The listing builds one solid part. Answer for the finished solid, in the listing's coordinates (mm). Coordinates: 2 decimals unless noted, no trailing zeros. Order: outer loops, then holes, each group sorted by start corner. A loop starts at its lowest first (then second) coordinate and runs counter-clockwise, first axis right, second up.
from build123d import *

# Parameters (mm, degrees)
SKETCH3_W           = 457.2
SKETCH3_H           = 609.6
BOSS_EXTRUDE1_DEPTH = 3.175
FILLET1_R           = 6.35


with BuildPart() as part:
    # Sketch3 → Boss-Extrude1 (new body)
    with BuildSketch(Plane(origin=(0, 0, 0), x_dir=(0, 0.3173046564050865, -0.9483236552062013), z_dir=(0, -0.9483236552062012, -0.3173046564050864))):
        Rectangle(SKETCH3_W, SKETCH3_H)
        with BuildLine():
            Line((203.2, -277.283333333), (177.8, -277.283333333))
            ThreePointArc((177.8, -277.283333333), (171.45, -270.933333333), (177.8, -264.583333333))
            Line((177.8, -264.583333333), (203.2, -264.583333333))
            ThreePointArc((203.2, -264.583333333), (209.55, -270.933333333), (203.2, -277.283333333))
        make_face(mode=Mode.SUBTRACT)
        with BuildLine():
            Line((-203.2, -264.583333333), (-177.8, -264.583333333))
            ThreePointArc((-177.8, -264.583333333), (-171.45, -270.933333333), (-177.8, -277.283333333))
            Line((-177.8, -277.283333333), (-203.2, -277.283333333))
            ThreePointArc((-203.2, -277.283333333), (-209.55, -270.933333333), (-203.2, -264.583333333))
        make_face(mode=Mode.SUBTRACT)
        with BuildLine():
            Line((203.2, 277.283333333), (177.8, 277.283333333))
            ThreePointArc((177.8, 277.283333333), (171.45, 270.933333333), (177.8, 264.583333333))
            Line((177.8, 264.583333333), (203.2, 264.583333333))
            ThreePointArc((203.2, 264.583333333), (209.55, 270.933333333), (203.2, 277.283333333))
        make_face(mode=Mode.SUBTRACT)
        with BuildLine():
            Line((-203.2, 264.583333333), (-177.8, 264.583333333))
            ThreePointArc((-177.8, 264.583333333), (-171.45, 270.933333333), (-177.8, 277.283333333))
            Line((-177.8, 277.283333333), (-203.2, 277.283333333))
            ThreePointArc((-203.2, 277.283333333), (-209.55, 270.933333333), (-203.2, 264.583333333))
        make_face(mode=Mode.SUBTRACT)
    extrude(amount=-BOSS_EXTRUDE1_DEPTH)

    # Fillet1
    fillet1_edges = [part.edges().sort_by_distance(p)[0] for p in [
        (-304.8, 74.041308257, -216.283066438),
        (-304.8, -71.030380652, 217.290508722),
        (304.8, -71.030380652, 217.290508722),
        (304.8, 74.041308257, -216.283066438),
    ]]
    fillet(fillet1_edges, radius=FILLET1_R)


solid = part.part
1) Each of these flat-tipped pins is pushed along its axis until it touches: P1, Ø12, axis at x = 27, z = 70, coming from the +Y side; P2, Ø1, axis at x = 54, z = -44.5, coming from the +Y side; P3, Ø2, axis at x = 147.5, z = -38.5, coming from the +Y side. Where does it stop, or does it pass through?
2) Section B-B (x = -7) is taken. Give the vertices of the cut face in (y, z), then the cut area to 3 significant figures.
3) Section A-A (z = -180) is taken. Give the vertices of the cut face in (x, y), then the cut area to 3 significant figures.
4) Consider L1, parallel to Y at x = -208, z = -113.5; L2, parallel to Y at x = 182, z = 141. Determine where each line is inside the solid, lowest interval first.
5) Section C-C (y = -28.5) is taken. Give the vertices of the cut face in (x, z), then the cut area to 3 significant figures.
Filled sheet:
1. P1: stops at y = -18.07
1. P2: stops at y = 18.4
1. P3: stops at y = 16.56
2. outline: (-72.54, 216.79) - (72.54, -216.79) - (75.55, -215.78) - (-69.52, 217.79) - close
2. area: 1,450 mm2
3. outline: (-304.8, 60.23) - (-277.28, 60.23) - (-277.28, 63.58) - (-304.8, 63.58) - close; (-264.58, 60.23) - (264.58, 60.23) - (264.58, 63.58) - (-264.58, 63.58) - close; (277.28, 60.23) - (304.8, 60.23) - (304.8, 63.58) - (277.28, 63.58) - close
3. area: 1,960 mm2
4. L1: y = 37.98 to 41.32
4. L2: y = -47.18 to -43.83
5. outline: (-304.8, 85.18) - (304.8, 85.18) - (304.8, 95.18) - (-304.8, 95.18) - close
5. area: 6,100 mm2
